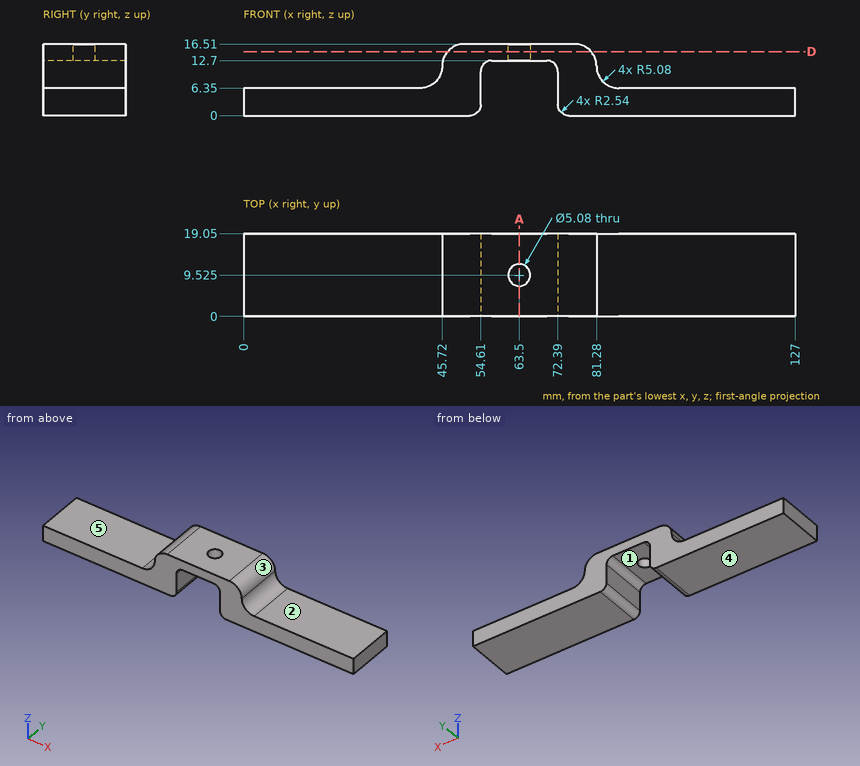
Design review of the part shown in the three views and the two pictorial views. Dimensions are in mm from the part's minimum x, y and z. A direction names the side the tool comes from. Round coordinates to 2 decimals unless told otherwise and drop trailing zeros. Order: outer loops, then holes, each group sorted by start corner. A loop starts at its lowest first (then second) coordinate and runs counter-clockwise, first axis right, second up.
Item 1: To check wall thickness, follow probe 1 along X at (y, z) = (10.25, 4.5); probe 2 along Y at (x, z) = (63.5, 14.65) (3 decimals); probe 3 along Z at (x, y) = (22, 11). State the ranges of each line that lie inside material, in increasing order.
Working result:
probe 1: x = 0 to 54.61, 72.39 to 127
probe 2: y = 0 to 6.985, 12.065 to 19.05
probe 3: z = 0 to 6.35
Item 2: Draft analysis for pull direction X (two halves, no side actions). For the marked faces 1, 2 and 3, state which applies: released by +X, released by -X, zero draft, split by the parting line, or undercut.
Working result:
face 1: undercut
face 2: zero draft
face 3: released by +X
Item 3: Machinability: for the marked faces 4 and 5, which of the approach directions +Z, -Z, +X, -X, +Y, -Y give a long, thin tool a straight path to every point of the face, cutting with its end or side? Answer none if there is none.
Working result:
face 4: -Z, +X, -X, +Y, -Y
face 5: +Z, -X, +Y, -Y
Item 4: For pin 1 (6 mm diameter, centred on y = 8.5, z = 10, fed in from +X); pin 2 (6 mm diameter, centred on y = 13, z = 11, fed in from +X); pin 3 (5.5 mm diameter, centred on x = 109, y = 10, fed in from +Z); pin 4 (8.5 mm diameter, centred on y = 8.5, z = 6.5, fed in from +X), all flat-tipped, find the tip position at first contact; note any pin that passes through.
Working result:
pin 1: stops at x = 83.87
pin 2: stops at x = 82.61
pin 3: stops at z = 6.35
pin 4: stops at x = 127
Item 5: Add section D-D, the plane z = 14.75. State the section outline as (x, y) points (3 decimals), and give its area (3 significant figures).
Working result:
outline: (46.955, 0) - (80.045, 0) - (80.045, 19.05) - (46.955, 19.05) - close; hole circle Ø5.08 at (63.5, 9.525)
area: 610 mm2
Item 6: Add section A-A, the plane x = 63.5. State the section outline as (y, z) points (3 decimals), and give its area (3 significant figures).
Working result:
outline: (0, 12.7) - (6.985, 12.7) - (6.985, 16.51) - (0, 16.51) - close; (12.065, 12.7) - (19.05, 12.7) - (19.05, 16.51) - (12.065, 16.51) - close
area: 53.2 mm2
